```python
from build123d import *

# Parameters (mm, degrees)
SKETCH011_W           = 6
SKETCH011_H           = 30
POCKET001_DEPTH       = 97.441731
POLARPATTERN001_COUNT = 5


with BuildPart() as part:
    # Sketch010 → Revolution003 (revolve)
    with BuildSketch(Plane.XZ):
        Polygon((-9.75, -10), (-9.75, 20), (-10.2, 20), (-11, 0), (-11, -10), align=None)
    revolve(axis=Axis((0, 0, 0), (0, 0, 1)))

    # Sketch011 → Pocket001 (cut, through all)
    with BuildSketch(Plane.XZ):
        with Locations((0, 15)):
            Rectangle(SKETCH011_W, SKETCH011_H)
    pocket001 = extrude(amount=-POCKET001_DEPTH, mode=Mode.SUBTRACT)

    # PolarPattern001: Pocket001 ×5 about axis
    polarpattern001_axis = Axis((0, 0, 0), (0, 0, 1))
    for i in range(1, POLARPATTERN001_COUNT):
        add(pocket001.rotate(polarpattern001_axis, i * 360 / POLARPATTERN001_COUNT), mode=Mode.SUBTRACT)


solid = part.part
```
Geometry: final body of the model. Coordinates: model frame, mm. A direction names the side the tool comes from. Coordinates: 2 decimals unless noted, no trailing zeros. Write each loop counter-clockwise with the first axis right and the second up, starting at its lowest first coordinate (ties: lowest second). Pieces come first, ordered by that corner, then holes. Notation, with made-up numbers: M 59.25,-32.75 L 98.25,-32.75 A15 ccw 98.25,-24.75 Z; hole C 26.5,44.5 d5. An arc over 180 degrees is marked long. Use CSV: the item, a comma, the result in double quotes. Start each with the question number.
1. Mould query, pull axis Y, two halves, no side actions, for faces 6 (the face through (-9.5, -3, 20)), 7 (the face through (6.276, 8.549, 9.86)), 8 (the face through (-3.319, -9.672, 7.638)). Classes: pulls with the +Y half, pulls with the -Y half, needs draft (parallel to the pull), parting line crosses it, or undercut.
2. Cut plane A-A on x = 0. Return the cut outline in (y, z), plus the area to 3 significant figures.
3. Ray query, probe 1 along X at (y, z) = (9.75, 1); probe 2 along X at (y, z) = (-4.25, 10.5); probe 3 along Y at (x, z) = (0, 7.25). Return the intervals inside material, ascending.
4. Cut plane B-B on y = 1. Return the cut outline in (x, z), plus the area to 3 significant figures.
5. Reachability of faces 1 (the face through (0, 10, 0)), 2 (the face through (-8.37, 5.874, 7.638)), 3 (the face through (8.173, -6.145, 7.638)), 4 (the face through (0, -10, 20)), 5 (the face through (8.37, 5.874, 7.638)) from +Z, -Z, +X, -X, +Y, -Y: full face, straight path, thin tool, end or side. Return the list, or none.
6. First-contact query: P1, Ø0.9, axis at x = -0.5, y = 10, coming from the +Z side; P2, Ø6, axis at x = 4.5, z = 0.5, coming from the -Y side; P3, Ø11.5, axis at x = 0, y = 0, coming from the -Z side; P4, Ø8, axis at x = 5, z = 16.5, coming from the -Y side. Flat tips, straight axial feed; report the tip coordinate or a pass-through.
7. Cut plane D-D on z = -8. Return the cut outline in (x, y), plus the area to 3 significant figures.
Entries:
1,face 6,"needs draft"
1,face 7,"pulls with the +Y half"
1,face 8,"undercut"
2,outline,"M -11,-10 L -9.75,-10 L -9.75,20 L -10.2,20 L -11,0 Z; M 9.75,-10 L 11,-10 L 11,0 L 9.75,0 Z"
2,area,"42.0 mm²"
3,probe 1,"-5.01 to -3, 3 to 5.01"
3,probe 2,"-9.69 to -8.77, 8.77 to 9.69"
3,probe 3,"-10.71 to -9.75"
4,outline,"M -10.95,-10 L -9.7,-10 L -9.7,0 L -10.95,0 Z; M 9.7,-10 L 10.95,-10 L 10.95,0 L 9.7,0 Z"
4,area,"25.1 mm²"
5,face 1,"+Z, +Y"
5,face 2,"+Z, -X"
5,face 3,"+Z, -Y"
5,face 4,"+Z, +X, -X, +Y, -Y"
5,face 5,"+Z, +X"
6,P1,"z = 0"
6,P2,"y = -10.89"
6,P3,"through"
6,P4,"y = -10.32"
7,outline,"C 0,0 d22; hole C 0,0 d19.5"
7,area,"81.5 mm²"
